Verification items for this drawing (mm, ordinates from the low corner). Give positions to 0.01 mm unless a question says otherwise; leave off trailing zeros. Write each loop counter-clockwise with the first axis right and the second up, starting at its lowest first coordinate (ties: lowest second). Pieces come first, ordered by that corner, then holes. Notation, with made-up numbers: (50.5, 56) -> (76.5, 56) arc R25 ccw to (76.5, 80) -> close; hole circle Ø9 at (68.25, 24). An arc over 180 degrees is marked (long way). Use one line per item in the form item = value. Start each with the question number.
(1) Section check C-C, the plane y = 138. Record the cut outline in (x, z), plus the area to 3 significant figures.
(2) Section check A-A, the plane y = 8. Record the cut outline in (x, z), plus the area to 3 significant figures.
(3) Scan lines: L1, parallel to Y at x = 113, z = 1.4; L2, parallel to X at y = 117, z = 2.2; L3, parallel to Y at x = 202, z = 2.95. Record each from-to range of solid material in increasing order.
(4) Section check B-B, the plane z = 3.75. Record the cut outline in (x, y).
(5) Depth check by flat-ended pin: pin 1 Ø2 at (x, z) = (157.5, 3) entering from -Y; pin 2 Ø3 at (y, z) = (81.5, 4) entering from -X; pin 3 Ø2.5 at (x, z) = (16.5, 3) entering from +Y. Enter the tip coordinate at first touch or a pass-through.
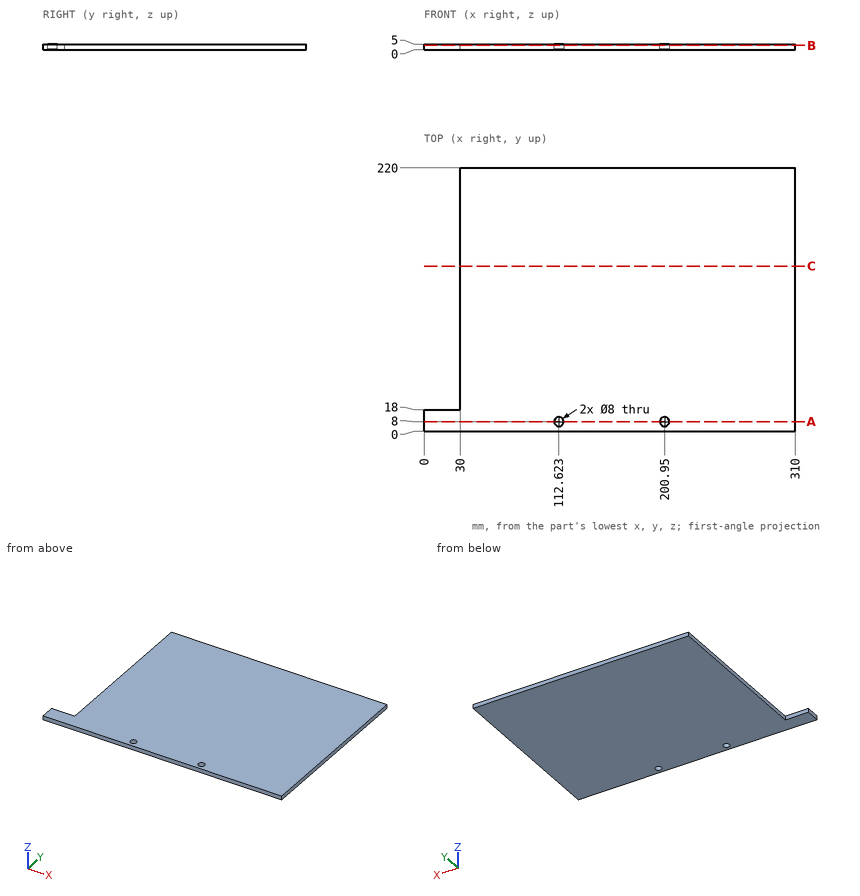
Completed:
q1.outline = (30, 0) -> (310, 0) -> (310, 5) -> (30, 5) -> close
q1.area = 1,400 mm²
q2.outline = (0, 0) -> (108.62, 0) -> (108.62, 5) -> (0, 5) -> close; (116.62, 0) -> (196.95, 0) -> (196.95, 5) -> (116.62, 5) -> close; (204.95, 0) -> (310, 0) -> (310, 5) -> (204.95, 5) -> close
q2.area = 1,470 mm²
q3.L1 = 0 to 4.02, 11.98 to 220
q3.L2 = 30 to 310
q3.L3 = 0 to 4.14, 11.86 to 220
q4.outline = (0, 0) -> (310, 0) -> (310, 220) -> (30, 220) -> (30, 18) -> (0, 18) -> close; hole circle Ø8 at (112.62, 8); hole circle Ø8 at (200.95, 8)
q5.pin_1 = 0
q5.pin_2 = 30
q5.pin_3 = 18
